Source: CAD feature listing. Evaluate the final solid. Frame: model axes, mm. A direction names the side the tool comes from. Give positions to 0.01 mm unless a question says otherwise; leave off trailing zeros. Loops run counter-clockwise (first coordinate to the right, second up) from the corner with the lowest first, then second, coordinate; pieces in that order, holes last.
Autodesk Inventor part; units mm, degrees
ref_plane "YZ Plane" through (0, 0, 0) normal (1, 0, 0) x (0, 1, 0)
ref_plane "XZ Plane" through (0, 0, 0) normal (0, 1, 0) x (-1, 0, 0)
ref_plane "XY Plane" through (0, 0, 0) normal (0, 0, 1) x (1, 0, 0)
sketch "Esquisse1" plane through (0, 0, 0) normal (1, 0, 0) x (0, 1, 0)
  line L0 (0, 0) -> (0, -31.2712)
  line L1 (18.75, -48) -> (18.75, -138)
  line L2 (18.75, -138) -> (0, -138)
  line L3 (14.75, -134) -> (14.75, -72.9524)
  line L4 (14.75, -72.9524) -> (7, -29)
  line L5 (7, -29) -> (7, -19)
  line L6 (7, -19) -> (8, -19)
  line L7 (8, -19) -> (9.7, -20.2)
  line L8 (9.7, -20.2) -> (10.85, -16.8246)
  line L9 (10.85, -16.8246) -> (8.25, -16)
  circle A0 centre (8.85, -17.7639) radius 1.5 construction
  line L10 (8.25, -16) -> (8.25, -5)
  line L11 (8.25, -5) -> (11.75, 0)
  line L12 (18.75, -48) -> (12.25, -48)
  line L13 (12.25, -48) -> (12.25, 0)
  line L14 (12.25, 0) -> (11.75, 0)
  line L15 (0, -138) -> (0, -134)
  line L16 (14.75, -134) -> (0, -134)
  point P0 (9.7477, -44.583)
  dimension "d1" = 37.5
  dimension "d3" = 14
  dimension "d6" = 3
  dimension "d7" = 10
  dimension "d8" = 1
  dimension "d11" = 3
  dimension "d12" = 0.6
  dimension "d13" = 1.2
  dimension "d14" = 1.7
  dimension "d15" = 2.6
  dimension "d29" = 24.5
  dimension "d30" = 0.5
  dimension "d31" = 48
  dimension "d34" = 11
  dimension "d36" = 16.5
  dimension "d37" = 19
  dimension "d38" = 90
  dimension "d58" = 7.75
  dimension "d59" = 170
  dimension "d60" = 19.4954
  dimension "d61" = 4
  dimension "d62" = 4
revolve "Révolution2" add sketch "Esquisse1" angle 360 about axis through (0, 0, 0) along (0, 0, -1)
sketch "Esquisse2" plane through (0, 0, 0) normal (0, 1, 0) x (-1, 0, 0)
  line L0 (-18.75, -48) -> (18.75, -48)
  line L1 (-18.75, -138) -> (18.75, -138)
  line L2 (-14.75, -72.9524) -> (14.75, -72.9524)
  line L3 (-7, -29) -> (7, -29)
  line L4 (-18.75, -48) -> (-18.75, -138)
  line L5 (-18.75, -60.7677) -> (-16.25, -59.8578)
  line L6 (-16.25, -59.8578) -> (-16.25, -64.1422)
  line L7 (-16.25, -64.1422) -> (-18.75, -63.2323)
  circle A0 centre (-17.75, -62) radius 1.5 construction
  line L8 (0, -168) -> (0, 28)
  point P0 (0, 0)
  dimension "d42" = 3
  dimension "d45" = 1
  dimension "d46" = 70
  dimension "d47" = 70
  dimension "d48" = 14
revolve "Révolution3" cut sketch "Esquisse2" angle 360 about axis through (0, 0, -10) along (0, 0, 1) contours L5 L6 L7 L4
chamfer "Chanfrein4" distance 1.5 angle 45 1 edges at (0, -12.25, -48)
pattern_linear "Réseau rectangulaire1" count 2 spacing 60 along (0, 0, -1) of "Révolution3"
chamfer "Chanfrein5" distance 2 angle 45 1 edges at (0, -14.75, -134)
sketch "Esquisse3" plane through (0, 0, 0) normal (0, 0, 1) x (1, 0, 0)
  circle A0 centre (0, 0) radius 11.75
  circle A1 centre (0, 0) radius 12.25
  line L0 (-1, 14.2091) -> (1, 14.2091)
  line L1 (1, 14.2091) -> (1, 12.2091)
  line L2 (1, 12.2091) -> (-1, 12.2091)
  line L3 (-1, 12.2091) -> (-1, 14.2091)
  circle A2 centre (0, 0) radius 12.25
  point P0 (0, 12.2091)
  dimension "d66" = 2
  dimension "d67" = 2
extrude "Extrusion1" add sketch "Esquisse3" against normal up to surface (48 mm away) contours L2 A1 | A1 L3 L0 L1 picked at (-0.1112, 12.2212)
chamfer "Chanfrein6" distance 0.5 angle 45 2 edges at (1, 14.2091, -24) (-1, 14.2091, -24)
sketch "Esquisse8" plane through (0, 0, -138) normal (0, 0, -1) x (-1, 0, 0)
  circle A0 centre (0, 0) radius 5
  dimension "d100" = 10
extrude "Extrusion5" cut sketch "Esquisse8" against normal up to surface (4 mm away)
chamfer "Chanfrein8" distance 1 angle 45 2 edges at (5, 0, -138) (5, 0, -134)
sketch "Esquisse9" plane through (0, 0, 0) normal (0, 1, 0) x (-1, 0, 0)
  line L0 (1, 0) -> (1, -46.5)
  line L1 (-1, -46.5) -> (1, -46.5)
  line L2 (-1, -46.5) -> (-1, 0)
  line L3 (-1, 0) -> (1, 0)
  line L4 (8.25, -5) -> (11.75, 0)
  line L5 (-8.25, -5) -> (-11.75, 0)
  line L6 (12.25, 0) -> (-12.25, 0)
  line L7 (-12.25, 0) -> (-12.25, -10)
  line L8 (-12.25, -10) -> (12.25, -10)
  line L9 (12.25, -10) -> (12.25, 0)
  line L10 (-12.25, 0) -> (12.25, 0)
  line L11 (-8.25, -5) -> (8.25, -5)
  line L12 (-12.25, 0) -> (-12.25, -46.5)
  point P0 (0, 0)
  dimension "d112" = 10
  dimension "d113" = 5
extrude "Extrusion6" cut sketch "Esquisse9" along normal blind 15 contours L6 L4 L11 L0 | L0 L11 L2 L3 | L11 L4 L6 L9 L8 L0 | L0 L8 L2 L11 | L2 L11 L5 L6 | L2 L8 L7 L6 L5 L11
chamfer "Chanfrein9" distance 2 angle 45 6 edges at (10, 0, -2.5) (-10, 0, -2.5) (8.25, 0, -7.5) (-8.25, 0, -7.5) (5.8336, 5.8336, -10) (-5.8336, 5.8336, -10)
sketch "Esquisse10" plane through (0, 0, 0) normal (0, 0, 1) x (1, 0, 0)
  arc A0 (-8.0064, -1.99) -> (8.0064, -1.99) centre (0, 0) ccw
  arc A1 (-11.5794, -1.9951) -> (11.5794, -1.9951) centre (0, 0) ccw
  arc A2 (-11.5794, -1.9951) -> (11.5794, -1.9951) centre (0, 0) ccw
  arc A3 (-12.1502, -1.5608) -> (12.1502, -1.5608) centre (0, 0) ccw
  line L0 (-2.75, -7.7782) -> (2.75, -7.7782)
  line L1 (2.75, -7.7782) -> (2.75, -12.25)
  line L2 (2.75, -12.25) -> (-2.75, -12.25)
  line L3 (-2.75, -12.25) -> (-2.75, -7.7782)
  arc A4 (-12.1502, -1.5608) -> (12.1502, -1.5608) centre (0, 0) ccw
  dimension "d114" = 5.5
extrude "Extrusion7" cut sketch "Esquisse10" against normal blind 13 contours A0 L1 A1 L3 | A1 L1 A3 L3 | A3 L2 L3 | L1 L2 A3
fillet "Congé1" radius 2 2 edges at (-2.75, -9.8578, -13) (2.75, -9.8578, -13)
chamfer "Chanfrein10" distance 1 angle 45 7 edges at (-2.75, -7.7782, -8) (-2.2552, -7.9358, -12.3169) (0, -8.25, -13) (2.2552, -7.9358, -12.3169) (2.75, -7.7782, -8) (-2.75, -9.4401, -2.7393) (2.75, -9.4401, -2.7393)
equation "\"d47\" = d46"
properties part number "douille_bloqueur"
(1) Mould query, pull axis Y, two halves, no side actions, for faces 6 (the conical face through (7.56, -6.59, -2.46)), 7 (the flat face through (-9, -8, 0)), 8 (the conical face through (12.569, -2.791, -133.875)). Classes: pulls with the +Y half, pulls with the -Y half, needs draft (parallel to the pull), parting line crosses it, or undercut.
A:
face 6: pulls with the +Y half
face 7: needs draft
face 8: undercut
(2) Reachability of faces 1 (the flat face through (2.75, -10, -7)), 2 (the cylindrical face through (18.59, -2.44, -92.4)), 3 (the cylindrical face through (15.5, -4.88, -62.03)), 4 (the flat face through (4.4, -4.4, -138)), 5 (the flat face through (-14, -1, -48)) from +Z, -Z, +X, -X, +Y, -Y: full face, straight path, thin tool, end or side. Return the list, or none.
A:
face 1: +Z, -Y
face 2: +Z, -Z
face 3: none
face 4: -Z, +X, -X, +Y, -Y
face 5: +Z
(3) First-contact query: pin 1 (2 mm diameter, centred on y = -7.5, z = -107, fed in from +X); pin 2 (0.8 mm diameter, centred on x = -0.5, y = -10, fed in from +Z); pin 3 (1.6 mm diameter, centred on x = -11, z = -6, fed in from +Y). Flat tips, straight axial feed; report the tip coordinate or a pass-through.
A:
pin 1: stops at x = 17.59
pin 2: stops at z = -12.99
pin 3: stops at y = 0
(4) Ray query, line 1 along X through (y, z) = (0, -90); line 2 along Z through (x, y) = (7, 15.5); line 3 along Y through (x, z) = (-10, -52). Return the intervals inside material, ascending.
A:
line 1: x = -18.75 to -14.75, 14.75 to 18.75
line 2: z = -138 to -123.87, -120.13 to -63.87, -60.13 to -48
line 3: y = -15.86 to -4.71, 4.71 to 15.86
(5) Section A-A, the plane z = -118. Return the cut outline in (x, y), then the cut area to 3 significant figures.
A:
outline: circle Ø37.5 at (0, 0); hole circle Ø29.5 at (0, 0)
area: 421 mm2
